Verification items for the finished model (mm, model axes). A direction names the side the tool comes from. Coordinates: 2 decimals unless noted, no trailing zeros. Order: outer loops, then holes, each group sorted by start corner. A loop starts at its lowest first (then second) coordinate and runs counter-clockwise, first axis right, second up. Notation, with made-up numbers: M -30.5,20.5 L -14.5,20.5 A20 cw -14.5,45.5 Z; hole C 52,-29.75 d8. An arc over 180 degrees is marked long. Return JSON: item names as keys, results as strings. Group by question number.
1. Gauge pin test, flat ends, axial feed: pin 1 (8 mm diameter, centred on x = 3.5, y = 5.5, fed in from -Z); pin 2 (1.5 mm diameter, centred on x = -12.5, z = -27, fed in from -Y); pin 3 (1.5 mm diameter, centred on x = -4.5, z = 61, fed in from +Y). Record the tip position at first contact, or that the pin passes through.
2. Section check A-A, the plane z = -16.5. Record the cut outline in (x, y), plus the area to 3 significant figures.
3. Material ranges on line 1 along Y through (x, z) = (0, 70); line 2 along Y through (x, z) = (0, -28); line 3 along Z through (x, y) = (0, -10), recorded low to high.
4. Section check D-D, the plane z = 68.5. Record the cut outline in (x, y), plus the area to 3 significant figures.
5. Section check B-B, the plane y = 8. Record the cut outline in (x, z).
6. Mould release check, pull along Y, two halves, no side actions. Record for faces 1 (the cylindrical face through (6.5, 12.4, 95.8)), 2 (the conical face through (0.481, 0.924, 100.475)), 3 (the flat face through (0, 0, 104.17)): +Y half, -Y half, draft (parallel to the pull), parting line (faces both ways), or undercut.
7. Section check C-C, the plane x = 11. Record the cut outline in (y, z).
8. Set-up check for faces 4 (the flat face through (4, 14, 87.17)), 5 (the cylindrical face through (-2.997, -9.667, 92.301)), 6 (the cylindrical face through (-3.47, 15.62, -13.67)): record each of +Z, -Z, +X, -X, +Y, -Y from which the full face is reachable in a straight line by a thin tool's end or side.
```python
from build123d import *

# Parameters (mm, degrees)
F2_R     = 3
F3_DEPTH = 25


with BuildPart() as f1:
    # F0 (on Front) → F1 (revolve)
    with BuildSketch(Plane.XZ):
        Polygon((16, 47.169506), (16, -72.830494), (21, -72.830494), (21, 87.169506), (14, 87.169506), (14, 97.169506), (14, 104.169506), (0, 104.169506), (0, 101.169506), (6, 97.169506), (6, 47.169506), align=None)
    revolve(axis=Axis((0, 0, -1.18644), (0, 0, -1)))

    # F2 (on Front) → F3 (cut, symmetric)
    with BuildSketch(Plane.XZ):
        with Locations((0, 92.169506)):
            Circle(F2_R)
    extrude(amount=F3_DEPTH, both=True, mode=Mode.SUBTRACT)


solid = f1.part
```
Answers follow:
{
 "1": {"pin 1": "z = 47.17", "pin 2": "y = -17.41", "pin 3": "y = 20.66"},
 "2": {"outline": "C 0,0 d42; hole C 0,0 d32", "area": "581 mm^2"},
 "3": {"line 1": "-21 to -6, 6 to 21", "line 2": "-21 to -16, 16 to 21", "line 3": "47.17 to 89.17, 95.17 to 104.17"},
 "4": {"outline": "C 0,0 d42; hole C 0,0 d12", "area": "1,270 mm^2"},
 "5": {"outline": "M -19.42,-72.83 L -13.86,-72.83 L -13.86,47.17 L 13.86,47.17 L 13.86,-72.83 L 19.42,-72.83 L 19.42,87.17 L 11.49,87.17 L 11.49,104.17 L -11.49,104.17 L -11.49,87.17 L -19.42,87.17 Z; hole C 0,92.17 d6"},
 "6": {"face 1": "parting line", "face 2": "undercut", "face 3": "draft"},
 "7": {"outline": "M -17.89,-72.83 L -11.62,-72.83 L -11.62,47.17 L 11.62,47.17 L 11.62,-72.83 L 17.89,-72.83 L 17.89,87.17 L 8.66,87.17 L 8.66,104.17 L -8.66,104.17 L -8.66,87.17 L -17.89,87.17 Z"},
 "8": {"face 4": "+Z", "face 5": "+Y, -Y", "face 6": "-Z"}
}
